from build123d import *

# Parameters (mm, degrees)
F0_W     = 1348.74
F0_H     = 685.8
F1_DEPTH = 25.4
F2_W     = 50.8
F2_H     = 76.2
F3_DEPTH = 711.2
F4_W     = 508
F4_H     = 25.4
F4_W_2   = 76.2
F5_DEPTH = 50.8
F6_W     = 355.6
F6_H     = 25.4
F6_W_2   = 76.2
F7_DEPTH = 50.8
F8_W     = 1348.74
F8_H     = 25.4
F9_DEPTH = 304.8
F10_R    = 12.7
F11_R    = 25.39999


# Not quite as in the source:
# - a fillet or chamfer is up to 0.001 mm smaller than in the source, because OpenCascade refuses the exact size


with BuildPart() as f1:
    # F0 (on Top) → F1 (new body)
    with BuildSketch(Plane.XY):
        Rectangle(F0_W, F0_H)
    extrude(amount=F1_DEPTH)

    # F2 (on face) → F3 (join)
    with BuildSketch(Plane.XY.offset(25.4)):
        with Locations((-648.97, 228.6)):
            Rectangle(F2_W, F2_H)
        with Locations((648.97, 228.6)):
            Rectangle(F2_W, F2_H)
    extrude(amount=-F3_DEPTH)

    # F4 (on face) → F5 (join)
    with BuildSketch(Plane(origin=(-674.37, 0, 0), x_dir=(0, -1, 0), z_dir=(-1, 0, 0))):
        with Locations((-88.9, -673.1)):
            Rectangle(F4_W, F4_H)
        with Locations((-304.8, -673.1)):
            Rectangle(F4_W_2, F4_H)
    extrude(amount=-F5_DEPTH)

    # F6 (on face) → F7 (join)
    with BuildSketch(Plane.YZ.offset(674.37)):
        with Locations((12.7, -673.1)):
            Rectangle(F6_W, F6_H)
        with Locations((228.6, -673.1)):
            Rectangle(F6_W_2, F6_H)
        with Locations((304.8, -673.1)):
            Rectangle(F6_W_2, F6_H)
    extrude(amount=-F7_DEPTH)

    # F8 (on face) → F9 (join)
    with BuildSketch(Plane(origin=(0, 0, 0), x_dir=(1, 0, 0), z_dir=(0, 0, -1))):
        with Locations((0, -254)):
            Rectangle(F8_W, F8_H)
    extrude(amount=F9_DEPTH)

    # F10
    f10_edges = [f1.edges().sort_by_distance(p)[0] for p in [
        (674.37, -342.9, 12.7),
        (-674.37, -342.9, 12.7),
        (-674.37, 342.9, 12.7),
        (674.37, 342.9, 12.7),
    ]]
    fillet(f10_edges, radius=F10_R)

    # F11 (radius 25.4 in the source; OpenCascade refuses exactly that, so slightly less here)
    f11_edges = [f1.edges().sort_by_distance(p)[0] for p in [
        (-623.57, -165.1, -673.1),
        (-674.37, -165.1, -673.1),
        (674.37, -165.1, -673.1),
        (623.57, -165.1, -673.1),
        (674.37, 342.9, -673.1),
        (623.57, 342.9, -673.1),
        (-674.37, 342.9, -673.1),
        (-623.57, 342.9, -673.1),
    ]]
    fillet(f11_edges, radius=F11_R)


solid = f1.part
CAD build for the part. Positions are in the model's coordinates, mm. A direction names the side the tool comes from. Round coordinates to 2 decimals unless told otherwise and drop trailing zeros. Order: outer loops, then holes, each group sorted by start corner. A loop starts at its lowest first (then second) coordinate and runs counter-clockwise, first axis right, second up. Notation, with made-up numbers: (84.25, 45.5) -> (97.25, 45.5) arc R30 ccw to (97.25, 70.5) -> close; hole circle Ø8 at (73, 12). An arc over 180 degrees is marked (long way). Write each question's results on one line, items separated by ' | '.
1. Wall check: line 1 along X through (y, z) = (224, -635); line 2 along Y through (x, z) = (-410.5, -38); line 3 along Z through (x, y) = (-230.5, -23.5). Give the ranges that are in metal, low to high. Write a range as [from, to].
Findings below:
line 1: x = [-674.37, -623.57], [623.57, 674.37] | line 2: y = [241.3, 266.7] | line 3: z = [0, 25.4]
2. Cut at C-C (x = 367). Give the cut face in (y, z), plus the area to 3 significant figures.
Findings below:
outline: (-342.9, 0) -> (241.3, 0) -> (241.3, -304.8) -> (266.7, -304.8) -> (266.7, 0) -> (342.9, 0) -> (342.9, 25.4) -> (-342.9, 25.4) -> close | area: 25,200 mm²
3. 3-axis set-ups, long thin cutter, end or side, ignore diameter. For faces 4 (the face through (-667.13, 335.26, -672.92)), 5 (the face through (-649, 190.5, -326)), 6 (the face through (-623.57, 192, -443)): which of +Z, -Z, +X, -X, +Y, -Y reach the whole face in a straight line?
Findings below:
face 4: -Z, -X, +Y | face 5: +X, -X, -Y | face 6: -Z, -Y
4. Cut at A-A (y = -28.5). Give the cut face in (x, z).
Findings below:
outline: (-674.37, -685.8) -> (-623.57, -685.8) -> (-623.57, -660.4) -> (-674.37, -660.4) -> close; (-674.37, 0) -> (674.37, 0) -> (674.37, 25.4) -> (-674.37, 25.4) -> close; (623.57, -685.8) -> (674.37, -685.8) -> (674.37, -660.4) -> (623.57, -660.4) -> close
5. Pull direction Z, two halves, no side cores. Call faces 1 (the face through (667.13, 335.26, -672.92)), 2 (the face through (-9, 5, 25.4)), 3 (the face through (649, 15, -660.4)): pulls with the +Z half, pulls with the -Z half, needs draft (parallel to the pull), parting line crosses it, or undercut.
Findings below:
face 1: needs draft | face 2: pulls with the +Z half | face 3: undercut
6. Cut at B-B (z = -627.5). Give the cut face in (x, y).
Findings below:
outline: (-674.37, 190.5) -> (-623.57, 190.5) -> (-623.57, 266.7) -> (-674.37, 266.7) -> close; (623.57, 190.5) -> (674.37, 190.5) -> (674.37, 266.7) -> (623.57, 266.7) -> close
7. Cut at D-D (z = -220). Give the cut face in (x, y), plus the area to 3 significant figures.
Findings below:
outline: (-674.37, 190.5) -> (-623.57, 190.5) -> (-623.57, 241.3) -> (623.57, 241.3) -> (623.57, 190.5) -> (674.37, 190.5) -> (674.37, 266.7) -> (-674.37, 266.7) -> close | area: 39,400 mm²
8. Flat gauge pins, fed straight in: P1, Ø15, axis at x = -643.5, z = -405, coming from the -Y side; P2, Ø10, axis at x = -397, z = -177.5, coming from the +Y side; P3, Ø3, axis at x = 371, z = -76.5, coming from the -Y side. Where does each tip first touch, or does it go through?
Findings below:
P1: stops at y = 190.5 | P2: stops at y = 266.7 | P3: stops at y = 241.3
